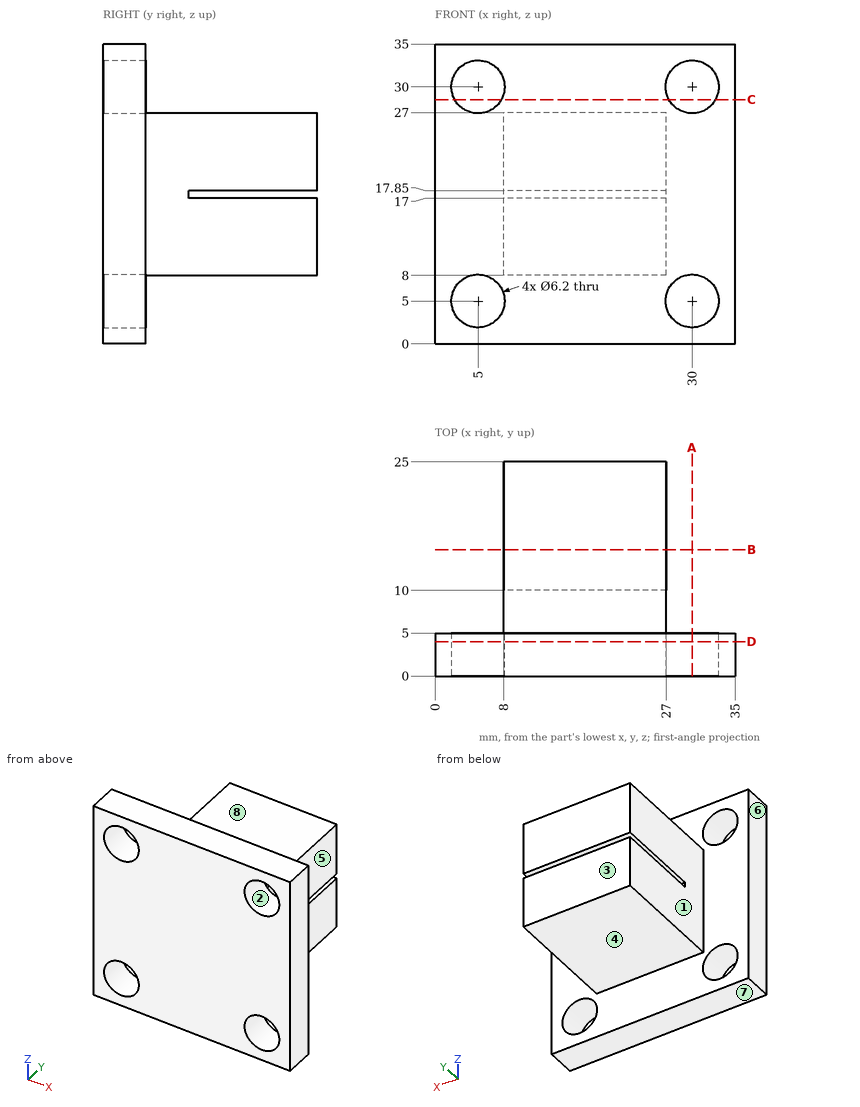
Geometry: see drawing. Coordinates: mm, zero at the bounding-box minimum. A direction names the side the tool comes from. Round coordinates to 2 decimals unless told otherwise and drop trailing zeros. Loops run counter-clockwise (first coordinate to the right, second up) from the corner with the lowest first, then second, coordinate; pieces in that order, holes last. Notation, with made-up numbers: (24.25, 79) - (81.25, 79) arc R26 cw to (81.25, 108) - close; hole circle Ø2 at (5, 14.25). An arc over 180 degrees is marked (long way). One line per item, written item: value. Start each with the question number.
(1) Section C-C, the plane z = 28.5. Return loops of the section in (x, y), plus the area to 3 significant figures.
(2) Access query for the marked faces 4, 5, 6, 7 and 8. Directions: +Z, -Z, +X, -X, +Y, -Y. A direction counts if a zero-diameter tool reaches every point of the face in a straight line with its end or side. Return the directions, or none.
(3) Contact query for flat-ended pins moving along their axis: P1, Ø12, axis at y = 19.5, z = 19.5, coming from the -X side; P2, Ø10, axis at x = 5, z = 30, coming from the -Y side; P3, Ø15, axis at y = 15, z = 19.5, coming from the +X side; P4, Ø7, axis at x = 30, z = 5, coming from the +Y side. Output: stop coordinate, or through.
(4) Section B-B, the plane y = 14.75. Return loops of the section in (x, z).
(5) Section A-A, the plane x = 30. Return loops of the section in (y, z).
(6) Section D-D, the plane y = 4. Return loops of the section in (x, z).
(7) Ray query, line 1 (Z direction, x = 5, y = 1.9); line 2 (Z direction, x = 17, y = 13.75); line 3 (Y direction, x = 5, z = 18). Return the intervals inside material, ascending. Write a range as [from, to].
(8) Draft query along X for the marked faces 1, 2 and 3. Return one class per face: +X half, -X half, draft (parallel to the pull), parting line (faces both ways), or undercut.
Results below:
1. outline: (0, 0) - (2.29, 0) - (2.29, 5) - (0, 5) - close; (7.71, 0) - (27.29, 0) - (27.29, 5) - (7.71, 5) - close; (32.71, 0) - (35, 0) - (35, 5) - (32.71, 5) - close
1. area: 121 mm^2
2. face 4: -Z, +X, -X, +Y
2. face 5: +Z, -Z, +X, +Y
2. face 6: +Z, -Z, -X, +Y, -Y
2. face 7: -Z, +X, -X, +Y, -Y
2. face 8: +Z, +X, -X, +Y
3. P1: x = 8
3. P2: y = 0
3. P3: x = 27
3. P4: y = 5
4. outline: (8, 8) - (27, 8) - (27, 17) - (8, 17) - close; (8, 17.85) - (27, 17.85) - (27, 27) - (8, 27) - close
5. outline: (0, 0) - (5, 0) - (5, 1.9) - (0, 1.9) - close; (0, 8.1) - (5, 8.1) - (5, 26.9) - (0, 26.9) - close; (0, 33.1) - (5, 33.1) - (5, 35) - (0, 35) - close
6. outline: (0, 0) - (35, 0) - (35, 35) - (0, 35) - close; hole circle Ø6.2 at (5, 5); hole circle Ø6.2 at (5, 30); hole circle Ø6.2 at (30, 5); hole circle Ø6.2 at (30, 30)
7. line 1: [0, 1.9], [8.1, 26.9], [33.1, 35]
7. line 2: [8, 17], [17.85, 27]
7. line 3: [0, 5]
8. face 1: -X half
8. face 2: undercut
8. face 3: draft
